The figure shows three views and two pictorial views of one solid part (mm, origin at its lowest corner). Answer the questions. A direction names the side the tool comes from. Coordinates: 2 decimals unless noted, no trailing zeros. Write each loop counter-clockwise with the first axis right and the second up, starting at its lowest first coordinate (ties: lowest second). Pieces come first, ordered by that corner, then holes.
Item 1: Each of these flat-tipped pins is pushed along its axis until it touches: P1, Ø1, axis at x = 0.5, y = 2.5, coming from the -Z side; P2, Ø2, axis at x = 4.5, z = 1.5, coming from the -Y side; P3, Ø2, axis at y = 5, z = 1.5, coming from the -X side; P4, Ø1.5, axis at y = 2, z = 5, coming from the +X side. Where does it stop, or does it pass through?
Item 2: Determine the mould class of the marked faces 1, 2 and 3 for opening direction Y: released by +Y, released by -Y, zero draft, split by the parting line, or undercut.
Item 3: Straight lines are drawn through the part: probe 1 along X at (y, z) = (2.95, 6); probe 2 along Z at (x, y) = (5.1, 4.6). For each, find the intervals that lie inside material, in ascending order.
Item 4: A tool of negligible diameter and unlimited length cuts with its end or side. For the marked faces 4 and 5, from which of +Z, -Z, +X, -X, +Y, -Y can it reach the whole face along a straight path? Write none if from no direction.
Item 5: Section C-C (z = 8.75) is taken. Give the vertices of the cut face in (x, y), then the cut area to 3 significant figures.
Item 6: Section A-A (y = 3) is taken. Give the vertices of the cut face in (x, z), then the cut area to 3 significant figures.
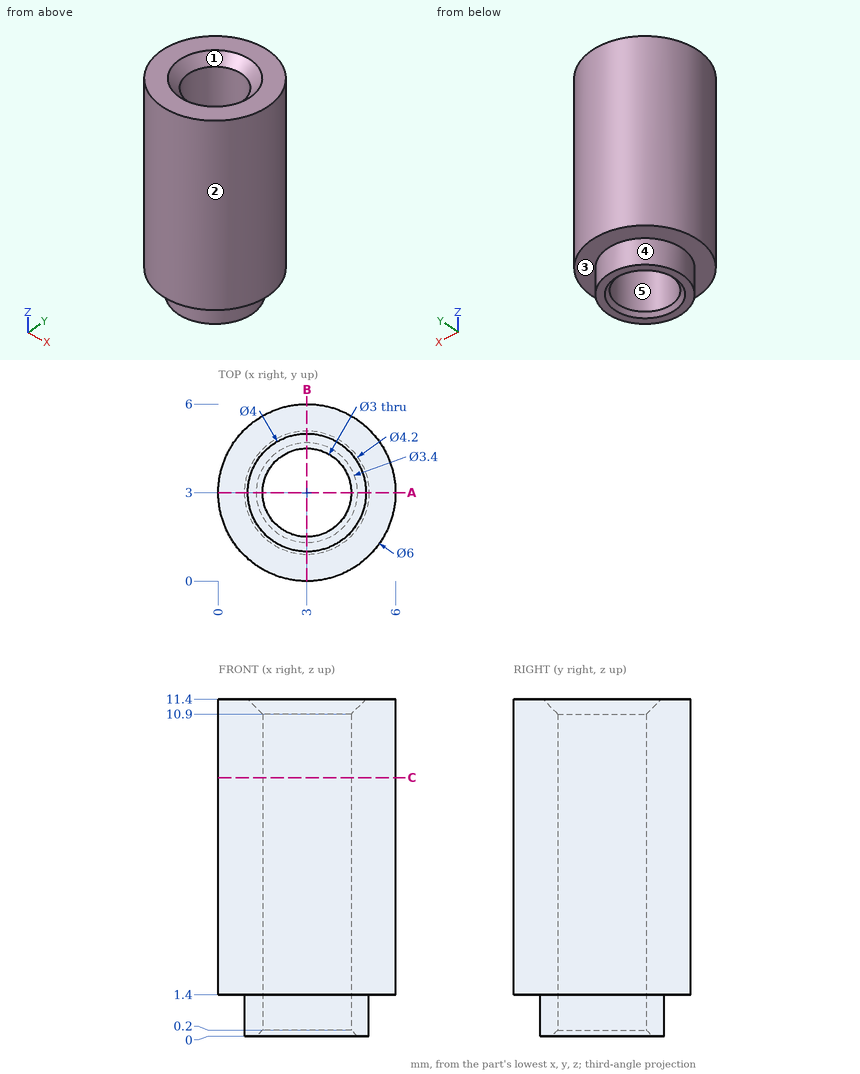
Established:
1. P1: stops at z = 0
1. P2: stops at y = 0.04
1. P3: stops at x = 0.17
1. P4: stops at x = 5.99
2. face 1: undercut
2. face 2: split by the parting line
2. face 3: zero draft
3. probe 1: x = 0 to 1.5, 4.5 to 6
3. probe 2: z = 1.4 to 11.4
4. face 4: -Z
4. face 5: +Z, -Z
5. outline: circle Ø6 at (3, 3); hole circle Ø3 at (3, 3)
5. area: 21.2 mm2
6. outline: (0, 1.4) - (0.9, 1.4) - (0.9, 0) - (1.3, 0) - (1.5, 0.2) - (1.5, 10.9) - (1, 11.4) - (0, 11.4) - close; (4.5, 0.2) - (4.7, 0) - (5.1, 0) - (5.1, 1.4) - (6, 1.4) - (6, 11.4) - (5, 11.4) - (4.5, 10.9) - close
6. area: 31.4 mm2
